Design review of the part built by this model. Coordinates are the model's own, in mm. Face numbers are marked on the shaded views. A direction names the side the tool comes from. Coordinates: 2 decimals unless noted, no trailing zeros. Loops run counter-clockwise (first coordinate to the right, second up) from the corner with the lowest first, then second, coordinate; pieces in that order, holes last. Notation, with made-up numbers: M 84.5,26.25 L 93.5,26.25 A25 cw 93.5,39.25 Z; hole C 28.25,32.25 d2. An arc over 180 degrees is marked long. Answer as a JSON object with one key per item and string values. Group by question number.
1. Insertion check: pin 1 (3 mm diameter, centred on y = 0.5, z = 3, fed in from +X); pin 2 (4 mm diameter, centred on x = -4, z = 1.5, fed in from +Y); pin 3 (2 mm diameter, centred on x = 2.5, z = 3.5, fed in from +Y). Each pin has a flat end and moves straight along its axis. Give the tip position at first contact, or say it passes through.
2. Consider section A-A (y = 0). State the section outline as (x, z) points, then the cut area to 3 significant figures.
3. Consider section D-D (y = 3.75). State the section outline as (x, z) points, then the cut area to 3 significant figures.
4. Draft analysis for pull direction Z (two halves, no side actions). For the marked faces 3, 4 and 5, state which applies: +Z half, -Z half, draft (parallel to the pull), parting line (faces both ways), or undercut.
5. To check wall thickness, follow probe 1 along Z at (x, y) = (3.75, 5); probe 2 along Y at (x, z) = (0, 4.75); probe 3 along X at (y, z) = (0.25, 3). State the ranges of each line that lie inside material, in increasing order.
6. Machinability: for the marked faces 1 and 2, which of the approach directions +Z, -Z, +X, -X, +Y, -Y give a long, thin tool a straight path to every point of the face, cutting with its end or side? Answer none if there is none.
7. Consider section C-C (z = 5). State the section outline as (x, y) points, then the cut area to 3 significant figures.
Autodesk Inventor part; units mm, degrees
ref_plane "YZ Plane" through (0, 0, 0) normal (1, 0, 0) x (0, 1, 0)
ref_plane "XZ Plane" through (0, 0, 0) normal (0, 1, 0) x (-1, 0, 0)
ref_plane "XY Plane" through (0, 0, 0) normal (0, 0, 1) x (1, 0, 0)
sketch "Sketch1" plane through (0, 0, 0) normal (0, 0, 1) x (1, 0, 0)
  circle A0 centre (0, 0) radius 6.75
  dimension "d0" = 13.5
extrude "Extrusion1" add sketch "Sketch1" along normal blind 1
sketch "Sketch2" plane through (0, 0, 1) normal (0, 0, 1) x (1, 0, 0)
  circle A0 centre (0, 0) radius 6.75
  circle A1 centre (0, 0) radius 5.5
  dimension "d3" = 11
extrude "Extrusion2" add sketch "Sketch2" along normal blind 6 contours A1
sketch "Sketch3" plane through (0, 0, 7) normal (0, 0, 1) x (1, 0, 0)
  circle A0 centre (0, 0) radius 5.5
  circle A1 centre (0, 0) radius 6.75
  dimension "d6" = 13.5
extrude "Extrusion3" add sketch "Sketch3" along normal blind 1 contours A0 | A1
sketch "Sketch4" plane through (0, 0, 8) normal (0, 0, 1) x (1, 0, 0)
  circle A0 centre (0, 0) radius 6.75
  circle A1 centre (0, 0) radius 2
  dimension "d9" = 4
extrude "Extrusion4" cut sketch "Sketch4" against normal blind 15 contours A1
properties material "Stainless Steel"
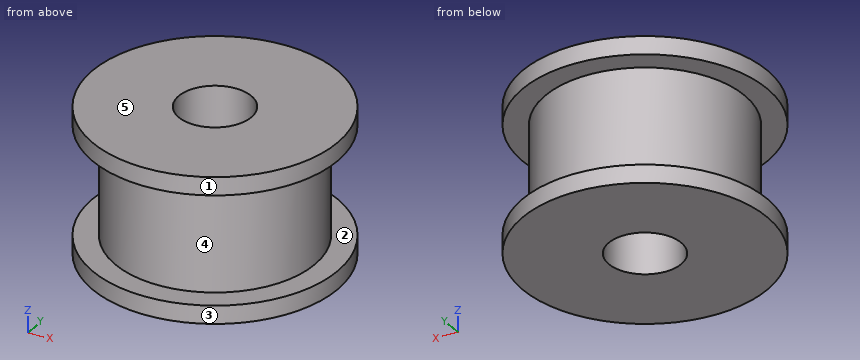
Findings below:
{
 "1": {"pin 1": "stops at x = 5.5", "pin 2": "stops at y = 6.43", "pin 3": "stops at y = 5.29"},
 "2": {"outline": "M -6.75,0 L -2,0 L -2,8 L -6.75,8 L -6.75,7 L -5.5,7 L -5.5,1 L -6.75,1 Z; M 2,0 L 6.75,0 L 6.75,1 L 5.5,1 L 5.5,7 L 6.75,7 L 6.75,8 L 2,8 Z", "area": "61.0 mm^2"},
 "3": {"outline": "M -5.61,0 L 5.61,0 L 5.61,1 L 4.02,1 L 4.02,7 L 5.61,7 L 5.61,8 L -5.61,8 L -5.61,7 L -4.02,7 L -4.02,1 L -5.61,1 Z", "area": "70.7 mm^2"},
 "4": {"face 3": "draft", "face 4": "undercut", "face 5": "+Z half"},
 "5": {"probe 1": "z = 0 to 1, 7 to 8", "probe 2": "y = -5.5 to -2, 2 to 5.5", "probe 3": "x = -5.49 to -1.98, 1.98 to 5.49"},
 "6": {"face 1": "+Z, -Z", "face 2": "none"},
 "7": {"outline": "C 0,0 d11; hole C 0,0 d4", "area": "82.5 mm^2"}
}
